Check sheet for the modelled part. Datum: model origin and axes. Units: mm. A direction names the side the tool comes from. Round coordinates to 2 decimals unless told otherwise and drop trailing zeros. Write each loop counter-clockwise with the first axis right and the second up, starting at its lowest first coordinate (ties: lowest second). Pieces come first, ordered by that corner, then holes.
Item 1: Set-up check for faces 1 (the flat face through (0, 0, 9)), 2 (the flat face through (0, -10, 6.985)): record each of +Z, -Z, +X, -X, +Y, -Y from which the full face is reachable in a straight line by a thin tool's end or side.
Item 2: Release check for a two-part mould opening along X. For faces 3 (the cylindrical face through (-9.08, -12.526, 8.326)), 4 (the cylindrical face through (-1.38, -22.27, -6.2)), 5 (the flat face through (5, -25.4, -5)) record: pulls with the +X half, pulls with the -X half, needs draft (parallel to the pull), parting line crosses it, or undercut.
Item 3: Section check B-B, the plane x = 0. Record the cut outline in (y, z) (3 decimals), plus the area to 3 significant figures.
Item 4: Material ranges on line 1 along Z through (x, y) = (0, -22.5); line 2 along Z through (x, y) = (-9, -9.75) (3 decimals); line 3 along Y through (x, z) = (6.5, -3.5), recorded low to high.
Item 5: Depth check by flat-ended pin: pin 1 (4 mm diameter, centred on x = -8, y = -18, fed in from +Z); pin 2 (12 mm diameter, centred on y = -7.5, z = -2, fed in from -X); pin 3 (2 mm diameter, centred on x = -3.5, y = -18, fed in from +Z). Enter the tip coordinate at first touch or a pass-through.
Item 6: Section check C-C, the plane z = 0. Record the cut outline in (x, y) (3 decimals), plus the area to 3 significant figures.
Item 7: Section check A-A, the plane y = -17.5. Record the cut outline in (x, z) (3 decimals).
Item 8: Section check D-D, the plane y = -22.25. Record the cut outline in (x, z).
from build123d import *

# Parameters (mm, degrees)
F0_R     = 12.319
F1_DEPTH = 25.4
F2_W     = 60.442776
F2_H     = 13.97
F3_DEPTH = 19.05
F4_R     = 6.35
F5_DEPTH = 25.4
F6_R     = 0.254


with BuildPart() as f1:
    # F0 (on Front) → F1 (new body)
    with BuildSketch(Plane.XZ):
        Circle(F0_R)
    extrude(amount=F1_DEPTH)

    # F2 (on face) → F3 (cut)
    with BuildSketch(Plane(origin=(0, 0, 0), x_dir=(-1, 0, 0), z_dir=(0, 1, 0))):
        Rectangle(F2_W, F2_H)
    extrude(amount=-F3_DEPTH, mode=Mode.SUBTRACT)

    # F4 (on face) → F5 (cut)
    with BuildSketch(Plane.XZ.offset(25.4)):
        Circle(F4_R)
    extrude(amount=-F5_DEPTH, mode=Mode.SUBTRACT)

    # F6
    f6_edges = [f1.edges().sort_by_distance(p)[0] for p in [
        (10.147292, -9.525, 6.985),
        (-10.147292, -9.525, 6.985),
        (0, 0, 6.985),
        (0, 0, 12.319),
        (0, 0, -12.319),
        (-10.147292, -9.525, -6.985),
        (10.147292, -9.525, -6.985),
        (0, 0, -6.985),
        (-12.319, -25.4, 0),
    ]]
    fillet(f6_edges, radius=F6_R)


solid = f1.part
Values found:
1. face 1: +Z, -Z, +X, -X, +Y
1. face 2: +X, -X, +Y
2. face 3: parting line crosses it
2. face 4: undercut
2. face 5: needs draft
3. outline: (-25.4, -12.065) arc R0.254 ccw to (-25.146, -12.319) - (-0.254, -12.319) arc R0.254 ccw to (0, -12.065) - (0, -7.239) arc R0.254 ccw to (-0.254, -6.985) - (-19.05, -6.985) - (-19.05, -6.35) - (-25.4, -6.35) - close; (-25.4, 6.35) - (-19.05, 6.35) - (-19.05, 6.985) - (-0.254, 6.985) arc R0.254 ccw to (0, 7.239) - (0, 12.065) arc R0.254 ccw to (-0.254, 12.319) - (-25.146, 12.319) arc R0.254 ccw to (-25.4, 12.065) - close
3. area: 279 mm2
4. line 1: z = -12.32 to -6.35, 6.35 to 12.32
4. line 2: z = -8.412 to -6.985, 6.985 to 8.412
4. line 3: y = -25.4 to -19.05
5. pin 1: stops at z = 10.76
5. pin 2: stops at x = -9.91
5. pin 3: stops at z = 12.06
6. outline: (-12.319, -25.146) arc R0.254 ccw to (-12.065, -25.4) - (-6.35, -25.4) - (-6.35, -19.05) - (-12.319, -19.05) - close; (6.35, -25.4) - (12.065, -25.4) arc R0.254 ccw to (12.319, -25.146) - (12.319, -19.05) - (6.35, -19.05) - close
6. area: 75.8 mm2
7. outline: (-9.855, -7.391) arc R12.319 ccw to (9.855, -7.391) arc R0.254 ccw to (9.652, -6.985) - (-9.652, -6.985) arc R0.254 ccw to start; (-9.855, 7.391) arc R0.254 ccw to (-9.652, 6.985) - (9.652, 6.985) arc R0.254 ccw to (9.855, 7.391) arc R12.319 ccw to start
8. outline: circle Ø24.64 at (0, 0); hole circle Ø12.7 at (0, 0)
